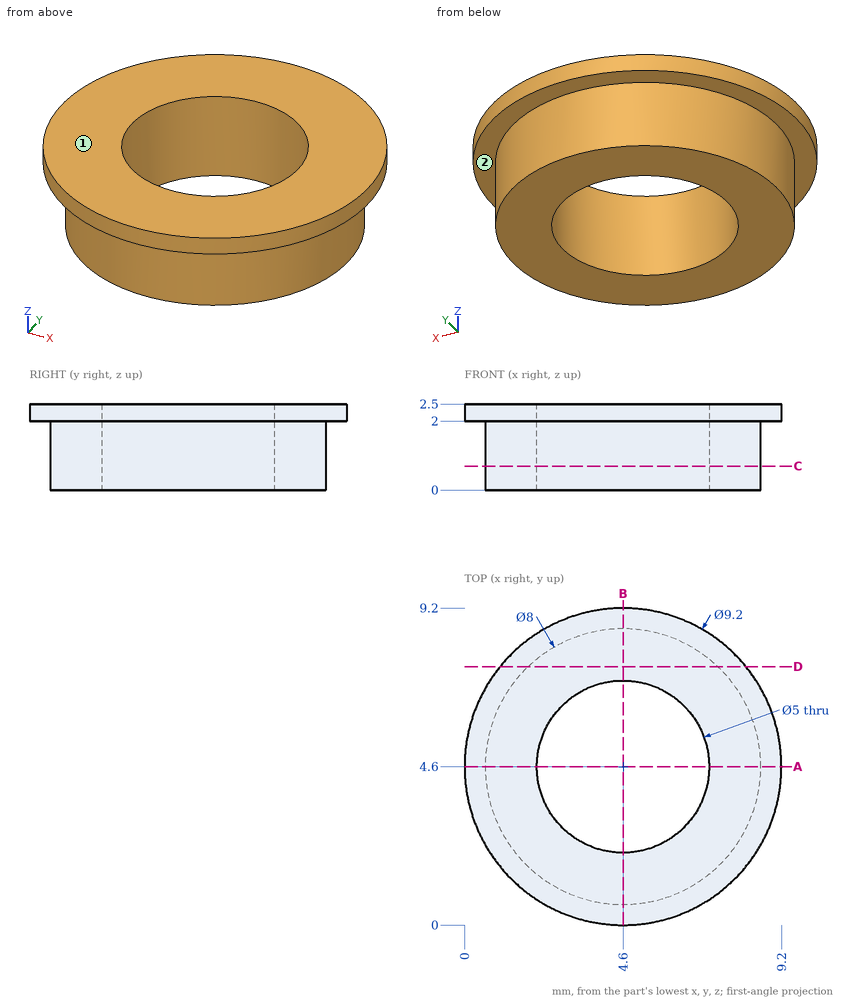
The figure shows three views and two pictorial views of one solid part (mm, origin at its lowest corner). Answer the questions. A direction names the side the tool comes from. Give positions to 0.01 mm unless a question says otherwise; leave off trailing zeros. Write each loop counter-clockwise with the first axis right and the second up, starting at its lowest first coordinate (ties: lowest second). Pieces come first, ordered by that corner, then holes. Notation, with made-up numbers: M 19,68.5 L 40,68.5 A20 ccw 40,85.5 Z; hole C 68.25,-40 d1. An arc over 180 degrees is marked long. One line per item, written item: value. Start each with the question number.
(1) Find section D-D (y = 7.5). Determine the outline of the cut face in (x, z) (3 decimals).
(2) A tool of negligible diameter and unlimited length cuts with its end or side. For the marked faces 1 and 2, from which of +Z, -Z, +X, -X, +Y, -Y can it reach the whole face along a straight path? Write none if from no direction.
(3) Find the intervals of material crossed by line 1 (X direction, y = 4.5, z = 1.1); line 2 (X direction, y = 5.5, z = 0.35), in increasing order.
(4) Find section C-C (z = 0.7). Determine the outline of the cut face in (x, y), plus the area to 3 significant figures.
(5) Find section A-A (y = 4.6). Determine the outline of the cut face in (x, z).
(6) Flat-ended cylindrical pins translate along their axes: pin 1 Ø1.5 at (x, z) = (3.5, 2) entering from -Y; pin 2 Ø3 at (x, y) = (2.5, 3) entering from -Z. Find the tip coordinate at first contact, or state that the pin passes through.
Results below:
1. outline: M 1.029,2 L 1.845,2 L 1.845,0 L 7.355,0 L 7.355,2 L 8.171,2 L 8.171,2.5 L 1.029,2.5 Z
2. face 1: +Z, +X, -X, +Y, -Y
2. face 2: -Z
3. line 1: x = 0.6 to 2.1, 7.1 to 8.6
3. line 2: x = 0.7 to 2.27, 6.93 to 8.5
4. outline: C 4.6,4.6 d8; hole C 4.6,4.6 d5
4. area: 30.6 mm^2
5. outline: M 0,2 L 0.6,2 L 0.6,0 L 2.1,0 L 2.1,2.5 L 0,2.5 Z; M 7.1,0 L 8.6,0 L 8.6,2 L 9.2,2 L 9.2,2.5 L 7.1,2.5 Z
6. pin 1: stops at y = 0.01
6. pin 2: stops at z = 0
